from build123d import *

# Parameters (mm, degrees)
F1_DEPTH = 8
F2_R     = 5
F3_R     = 1


with BuildPart() as f1:
    # F0 (on Top) → F1 (new body)
    with BuildSketch(Plane.XY):
        with BuildLine():
            Line((68.7570372224, 46.9683377401), (-61.2429627776, 46.9683377401))
            ThreePointArc((-61.2429627776, 46.9683377401), (-64.7784966835, 45.503871646), (-66.2429627776, 41.9683377401))
            Line((-66.2429627776, 41.9683377401), (-66.2429627776, -18.0316622599))
            ThreePointArc((-66.2429627776, -18.0316622599), (-64.7784966835, -21.5671961658), (-61.2429627776, -23.0316622599))
            Line((-61.2429627776, -23.0316622599), (68.7570372224, -23.0316622599))
            ThreePointArc((68.7570372224, -23.0316622599), (72.2925711283, -21.5671961658), (73.7570372224, -18.0316622599))
            Line((73.7570372224, -18.0316622599), (73.7570372224, 41.9683377401))
            ThreePointArc((73.7570372224, 41.9683377401), (72.2925711283, 45.503871646), (68.7570372224, 46.9683377401))
        make_face()
    extrude(amount=F1_DEPTH)

    # F2
    f2_edges = [f1.edges().sort_by_distance(p)[0] for p in [
        (3.757037, -23.031662, 0),
        (73.757037, 11.968338, 0),
    ]]
    fillet(f2_edges, radius=F2_R)

    # F3
    f3_edges = [f1.edges().sort_by_distance(p)[0] for p in [
        (3.757037, 46.968338, 8),
        (-64.778497, 45.503872, 8),
        (-66.242963, 11.968338, 8),
        (-64.778497, -21.567196, 8),
        (3.757037, -23.031662, 8),
        (72.292571, -21.567196, 8),
        (73.757037, 11.968338, 8),
        (72.292571, 45.503872, 8),
    ]]
    fillet(f3_edges, radius=F3_R)


solid = f1.part
Can you work these out from the model? Positions are in its coordinate system, mm. Give positions to 0.01 mm unless a question says otherwise; leave off trailing zeros. Order: outer loops, then holes, each group sorted by start corner. A loop starts at its lowest first (then second) coordinate and runs counter-clockwise, first axis right, second up. Notation, with made-up numbers: M 88.5,10.25 L 102.5,10.25 A19 ccw 102.5,21.25 Z; hole C 82.25,60 d3. An arc over 180 degrees is marked long. One line per question, with ' | ' between items.
Item 1: Please list where these lines run through material, in increasing order: L1, parallel to Y at x = 1.5, z = 4.75; L2, parallel to X at y = 42, z = 4.5; L3, parallel to Y at x = -59.5, z = 7.25.
Answer block:
L1: y = -23.03 to 46.96 | L2: x = -66.22 to 73.73 | L3: y = -23 to 46.94
Item 2: Suppose I cut it at A-A, the plane x = 47. Write out the boundary of the cut face in (y, z), then the cut area to 3 significant figures.
Answer block:
outline: M -23.03,5 A5 ccw -18.03,0 L 41.97,0 A5 ccw 46.97,5 L 46.97,7 A1 ccw 45.97,8 L -22.03,8 A1 ccw -23.03,7 Z | area: 549 mm2
Item 3: Suppose I cut it at B-B, the plane z = 3.25. Write out the boundary of the cut face in (x, y).
Answer block:
outline: M -65.93,-18.03 A4.68 ccw -61.24,-22.72 L 68.76,-22.72 A4.68 ccw 73.44,-18.03 L 73.44,41.97 A4.68 ccw 68.76,46.65 L -61.24,46.65 A4.68 ccw -65.93,41.97 Z
Item 4: I'm going to push a flat-ended pin straight in: pin 1 Ø1 at (y, z) = (2, 3) entering from -X. Where does the tip first touch, or does it pass through?
Answer block:
pin 1: stops at x = -66.01
